For this review, take the finished solid that the model builds, in its own axes (mm). Round coordinates to 2 decimals unless told otherwise and drop trailing zeros. Loops run counter-clockwise (first coordinate to the right, second up) from the corner with the lowest first, then second, coordinate; pieces in that order, holes last.
1. Consider section C-C on x = -2.75. State the section outline as (y, z) points.
2. Consider section A-A on y = 1. State the section outline as (x, z) points, then the cut area to 3 significant figures.
3. To check wall thickness, follow line 1 along X through (y, z) = (-2, 0.1); line 2 along X through (y, z) = (-1.5, 0.6); line 3 along Y through (x, z) = (0, 0.3). State the ranges of each line that lie inside material, in increasing order.
4. Consider section D-D on x = 0. State the section outline as (y, z) points, then the cut area to 3 significant figures.
5. Draft analysis for pull direction X (two halves, no side actions). For faces 1 (the cylindrical face through (0.1, 3.7, 0.3)), 2 (the cylindrical face through (-0.1, 2.4, 0.3)), 3 (the flat face through (0, 3, 0.7)), state which applies: released by +X, released by -X, zero draft, split by the parting line, or undercut.
6. Consider section B-B on z = 0.4. State the section outline as (x, y) points.
7. Clearance check with a flat-ended pin moving along its axis: pin 1 Ø2 at (x, y) = (-0.5, -1) entering from -Z. State where the tip first meets the part, or that it passes through.
from build123d import *

# Parameters (mm, degrees)
BOSS_EXTRUDE1_DEPTH = 0.7


with BuildPart() as part:
    # Sketch2 → Boss-Extrude1 (new body)
    with BuildSketch(Plane.XY):
        with BuildLine():
            Line((-2.156675683, -1.78877445), (-2.156675683, -1.420873217))
            Line((-2.156675683, -1.420873217), (-2.156675683, -1.052971984))
            ThreePointArc((-2.156675683, -1.052971984), (-2.233146653, -0.879236046), (-2.295648057, -0.7))
            ThreePointArc((-2.295648057, -0.7), (-2.71665879, -0.466883635), (-2.833333333, 0))
            ThreePointArc((-2.833333333, 0), (0, 2.4), (2.833333333, 0))
            ThreePointArc((2.833333333, 0), (2.71665879, -0.466883635), (2.295648057, -0.7))
            ThreePointArc((2.295648057, -0.7), (2.233146653, -0.879236046), (2.156675683, -1.052971984))
            Line((2.156675683, -1.052971984), (2.156675683, -1.420873217))
            Line((2.156675683, -1.420873217), (2.156675683, -1.78877445))
            ThreePointArc((2.156675683, -1.78877445), (2.248723901, -2.15372226), (2.463088621, -2.463088621))
            Line((2.463088621, -2.463088621), (2.61629509, -2.61629509))
            ThreePointArc((2.61629509, -2.61629509), (0, 3.7), (-2.61629509, -2.61629509))
            Line((-2.61629509, -2.61629509), (-2.463088621, -2.463088621))
            ThreePointArc((-2.463088621, -2.463088621), (-2.248723901, -2.15372226), (-2.156675683, -1.78877445))
        make_face()
    extrude(amount=BOSS_EXTRUDE1_DEPTH)


solid = part.part
Resolved:
1. outline: (-2.48, 0) - (-0.42, 0) - (-0.42, 0.7) - (-2.48, 0.7) - close; (0.36, 0) - (2.48, 0) - (2.48, 0.7) - (0.36, 0.7) - close
2. outline: (-3.56, 0) - (-2.47, 0) - (-2.47, 0.7) - (-3.56, 0.7) - close; (2.47, 0) - (3.56, 0) - (3.56, 0.7) - (2.47, 0.7) - close
2. area: 1.53 mm2
3. line 1: x = -3.11 to -2.19, 2.19 to 3.11
3. line 2: x = -3.38 to -2.16, 2.16 to 3.38
3. line 3: y = 2.4 to 3.7
4. outline: (2.4, 0) - (3.7, 0) - (3.7, 0.7) - (2.4, 0.7) - close
4. area: 0.910 mm2
5. face 1: split by the parting line
5. face 2: undercut
5. face 3: zero draft
6. outline: (-2.83, 0) arc R2.87 cw to (2.83, 0) arc R0.6 cw to (2.3, -0.7) arc R2.4 cw to (2.16, -1.05) - (2.16, -1.79) arc R1.05 ccw to (2.46, -2.46) - (2.62, -2.62) arc R3.7 ccw (long way) to (-2.62, -2.62) - (-2.46, -2.46) arc R1.05 ccw to (-2.16, -1.79) - (-2.16, -1.05) arc R2.4 cw to (-2.3, -0.7) arc R0.6 cw to start
7. pin 1: passes through
